Here's how the part is built. I have some questions about the finished solid (model axes, mm). A direction names the side the tool comes from. Coordinates: 2 decimals unless noted, no trailing zeros. Loops run counter-clockwise (first coordinate to the right, second up) from the corner with the lowest first, then second, coordinate; pieces in that order, holes last. Notation, with made-up numbers: (28, -9) - (74, -9) arc R27 ccw to (74, 29) - close; hole circle Ø9 at (10.5, -2). An arc over 180 degrees is marked (long way). Use a Markdown table: item, result.
```python
from build123d import *

# Parameters (mm, degrees)
BOSS_EXTRUDE1_DEPTH = 37
SKETCH2_R           = 1.75
SKETCH2_R_2         = 12.5
SKETCH2_R_3         = 2.75
SKETCH2_R_4         = 2.25
CUT_EXTRUDE1_DEPTH  = 38
SKETCH5_R           = 2.25
CUT_EXTRUDE2_DEPTH  = 38
CUT_EXTRUDE3_DEPTH  = 34
SKETCH7_R           = 4.75
BOSS_EXTRUDE2_DEPTH = 4.5
SKETCH10_W          = 40
SKETCH10_H          = 64
CUT_EXTRUDE4_DEPTH  = 34
SKETCH11_R          = 2.75
CUT_EXTRUDE5_DEPTH  = 8.5
SKETCH12_W          = 15
SKETCH12_H          = 10
SKETCH12_W_2        = 20
SKETCH12_W_3        = 10
BOSS_EXTRUDE3_DEPTH = 34
CUT_EXTRUDE6_DEPTH  = 33
CUT_EXTRUDE8_DEPTH  = 15
CUT_EXTRUDE9_DEPTH  = 15
CUT_EXTRUDE10_DEPTH = 10
CUT_EXTRUDE11_DEPTH = 10
SKETCH20_W          = 6
SKETCH20_H          = 15
CUT_EXTRUDE12_DEPTH = 3


with BuildPart() as part:
    # Sketch1 → Boss-Extrude1 (new body)
    with BuildSketch(Plane.XY):
        with BuildLine():
            Line((-78, 32), (78, 32))
            ThreePointArc((78, 32), (81.535533906, 30.535533906), (83, 27))
            Line((83, 27), (83, -27))
            ThreePointArc((83, -27), (81.535533906, -30.535533906), (78, -32))
            Line((78, -32), (-78, -32))
            ThreePointArc((-78, -32), (-81.535533906, -30.535533906), (-83, -27))
            Line((-83, -27), (-83, 27))
            ThreePointArc((-83, 27), (-81.535533906, 30.535533906), (-78, 32))
        make_face()
    extrude(amount=BOSS_EXTRUDE1_DEPTH)

    # Sketch2 → Cut-Extrude1 (cut, through all)
    with BuildSketch(Plane.XY.offset(37)):
        with Locations((-73.75, 15.75)):
            Circle(SKETCH2_R)
        with Locations((-42.25, 15.75)):
            Circle(SKETCH2_R)
        with Locations((-73.75, -15.75)):
            Circle(SKETCH2_R)
        with Locations((-42.25, -15.75)):
            Circle(SKETCH2_R)
        with Locations((-58, 0)):
            Circle(SKETCH2_R_2)
        with Locations((44, 15)):
            Circle(SKETCH2_R_3)
        with Locations((44, -15)):
            Circle(SKETCH2_R_3)
        with Locations((-18, 0)):
            Circle(SKETCH2_R_3)
        with Locations((64, 0)):
            Circle(SKETCH2_R_4)
    extrude(amount=-CUT_EXTRUDE1_DEPTH, mode=Mode.SUBTRACT)

    # Sketch5 → Cut-Extrude2 (cut, through all)
    with BuildSketch(Plane.XY.offset(37)):
        with Locations((3, 0)):
            Circle(SKETCH5_R)
        with Locations((23, 0)):
            Circle(SKETCH5_R)
    extrude(amount=-CUT_EXTRUDE2_DEPTH, mode=Mode.SUBTRACT)

    # Sketch6 → Cut-Extrude3 (cut)
    with BuildSketch(Plane.XY.offset(37)):
        with BuildLine():
            Line((-78, -29), (78, -29))
            ThreePointArc((78, -29), (79.414213562, -28.414213562), (80, -27))
            Line((80, -27), (80, 27))
            ThreePointArc((80, 27), (79.414213562, 28.414213562), (78, 29))
            Line((78, 29), (-78, 29))
            ThreePointArc((-78, 29), (-79.414213562, 28.414213562), (-80, 27))
            Line((-80, 27), (-80, -27))
            ThreePointArc((-80, -27), (-79.414213562, -28.414213562), (-78, -29))
        make_face()
    extrude(amount=-CUT_EXTRUDE3_DEPTH, mode=Mode.SUBTRACT)

    # Sketch7 → Boss-Extrude2 (add)
    with BuildSketch(Plane.XY.offset(3)):
        with Locations((-18, 0)):
            Circle(SKETCH7_R)
        with Locations((44, -15)):
            Circle(SKETCH7_R)
        with Locations((44, 15)):
            Circle(SKETCH7_R)
    extrude(amount=BOSS_EXTRUDE2_DEPTH)

    # Sketch10 → Cut-Extrude4 (cut)
    with BuildSketch(Plane.XY.offset(37)):
        with Locations((13, 0)):
            Rectangle(SKETCH10_W, SKETCH10_H)
    extrude(amount=-CUT_EXTRUDE4_DEPTH, mode=Mode.SUBTRACT)

    # Sketch11 → Cut-Extrude5 (cut, through all)
    with BuildSketch(Plane.XY.offset(7.5)):
        with Locations((44, -15)):
            Circle(SKETCH11_R)
        with Locations((-18, 0)):
            Circle(SKETCH11_R)
        with Locations((44, 15)):
            Circle(SKETCH11_R)
    extrude(amount=-CUT_EXTRUDE5_DEPTH, mode=Mode.SUBTRACT)

    # Sketch12 → Boss-Extrude3 (add, through all)
    with BuildSketch(Plane.XY.offset(3)):
        with Locations((67.5, -24)):
            Rectangle(SKETCH12_W, SKETCH12_H)
        with Locations((67.5, 24)):
            Rectangle(SKETCH12_W, SKETCH12_H)
        with Locations((70, -11)):
            Rectangle(SKETCH12_W_2, SKETCH12_H)
        with Locations((70, 11)):
            Rectangle(SKETCH12_W_2, SKETCH12_H)
        with Locations((-30, -24)):
            Rectangle(SKETCH12_W_3, SKETCH12_H)
        with Locations((-30, 24)):
            Rectangle(SKETCH12_W_3, SKETCH12_H)
    extrude(amount=BOSS_EXTRUDE3_DEPTH)

    # Sketch14 → Cut-Extrude6 (cut)
    with BuildSketch(Plane.XZ.offset(16)):
        Polygon((80, 37), (60, 37), (60, 3), align=None)
    extrude(amount=-CUT_EXTRUDE6_DEPTH, mode=Mode.SUBTRACT)

    # Sketch16 → Cut-Extrude8 (cut)
    with BuildSketch(Plane(origin=(75, 0, 0), x_dir=(0, 0, -1), z_dir=(1, 0, 0))):
        Polygon((-37, -19), (-3, -19), (-37, -29), align=None)
    extrude(amount=-CUT_EXTRUDE8_DEPTH, mode=Mode.SUBTRACT)

    # Sketch17 → Cut-Extrude9 (cut)
    with BuildSketch(Plane.ZY.offset(-60)):
        Polygon((37, 19), (3, 19), (37, 29), align=None)
    extrude(amount=-CUT_EXTRUDE9_DEPTH, mode=Mode.SUBTRACT)

    # Sketch18 → Cut-Extrude10 (cut)
    with BuildSketch(Plane(origin=(-25, 0, 0), x_dir=(0, 0, -1), z_dir=(1, 0, 0))):
        Polygon((-37, -29), (-37, -19), (-3, -19), align=None)
    extrude(amount=-CUT_EXTRUDE10_DEPTH, mode=Mode.SUBTRACT)

    # Sketch19 → Cut-Extrude11 (cut)
    with BuildSketch(Plane(origin=(-25, 0, 0), x_dir=(0, 0, -1), z_dir=(1, 0, 0))):
        Polygon((-37, 29), (-3, 19), (-37, 19), align=None)
    extrude(amount=-CUT_EXTRUDE11_DEPTH, mode=Mode.SUBTRACT)

    # Sketch20 → Cut-Extrude12 (cut)
    with BuildSketch(Plane.ZY.offset(83)):
        with Locations((30, 0)):
            Rectangle(SKETCH20_W, SKETCH20_H)
    extrude(amount=-CUT_EXTRUDE12_DEPTH, mode=Mode.SUBTRACT)


solid = part.part
```
Q1. I want a section at A-A, the plane x = -42.25. Write out the boundary of the cut face in (y, z), then the cut area to 3 significant figures.
Check values:
| item | result |
|---|---|
| outline | (-32, 0) - (-17.5, 0) - (-17.5, 3) - (-29, 3) - (-29, 37) - (-32, 37) - close; (-14, 0) - (14, 0) - (14, 3) - (-14, 3) - close; (17.5, 0) - (32, 0) - (32, 37) - (29, 37) - (29, 3) - (17.5, 3) - close |
| area | 375 mm^2 |
Q2. Will these pins go through, and if not, where does the flat tip stop? P1, Ø1, axis at x = 47.5, y = 21, coming from the +Z side; P2, Ø2.5, axis at x = -81, y = 3.5, coming from the -Z side.
Check values:
| item | result |
|---|---|
| P1 | z = 3 |
| P2 | z = 0 |
Q3. If we mould it in two halves opening along X, with no side actions, what happens to faces 1 (the face through (-16, -29, 20)), 2 (the face through (-82, 30, 18)), 3 (the face through (82, -30, 18))? For each: pulls with the +X half, pulls with the -X half, needs draft (parallel to the pull), parting line crosses it, or undercut.
Check values:
| item | result |
|---|---|
| face 1 | undercut |
| face 2 | pulls with the -X half |
| face 3 | pulls with the +X half |
Q4. Which directions (+Z, -Z, +X, -X, +Y, -Y) give clear straight access to the entire face, cutting with the end or side of a thin tool? Please do faces 4 (the face through (-35, 26, 12)), 5 (the face through (-82, -7.5, 30)), 6 (the face through (-40.581, -15.224, 1.521)).
Check values:
| item | result |
|---|---|
| face 4 | +Z |
| face 5 | -X |
| face 6 | +Z, -Z |
Q5. I want a section at D-D, the plane x = 44. Write out the boundary of the cut face in (y, z).
Check values:
| item | result |
|---|---|
| outline | (-32, 0) - (-17.75, 0) - (-17.75, 7.5) - (-19.75, 7.5) - (-19.75, 3) - (-29, 3) - (-29, 37) - (-32, 37) - close; (-12.25, 0) - (12.25, 0) - (12.25, 7.5) - (10.25, 7.5) - (10.25, 3) - (-10.25, 3) - (-10.25, 7.5) - (-12.25, 7.5) - close; (17.75, 0) - (32, 0) - (32, 37) - (29, 37) - (29, 3) - (19.75, 3) - (19.75, 7.5) - (17.75, 7.5) - close |
Q6. I want a section at C-C, the plane y = -24.5. Write out the boundary of the cut face in (x, z).
Check values:
| item | result |
|---|---|
| outline | (-83, 0) - (83, 0) - (83, 37) - (80, 37) - (80, 3) - (75, 3) - (75, 21.7) - (60, 21.7) - (60, 3) - (-25, 3) - (-25, 21.7) - (-35, 21.7) - (-35, 3) - (-80, 3) - (-80, 37) - (-83, 37) - close |
Q7. Please list where these lines run through material, in increasing order: L1, parallel to X at y = -21.5, z = 6.5; L2, parallel to Y at x = -42.25, z = 1; L3, parallel to X at y = 24, z = 22. Write a range as from..to.
Check values:
| item | result |
|---|---|
| L1 | -83..-80, -35..-25, 60..75, 80..83 |
| L2 | -32..-17.5, -14..14, 17.5..32 |
| L3 | -83..-80, 80..83 |
Q8. I want a section at B-B, the plane x = -18. Write out the boundary of the cut face in (y, z), then the cut area to 4 significant figures.
Check values:
| item | result |
|---|---|
| outline | (-32, 0) - (-2.75, 0) - (-2.75, 7.5) - (-4.75, 7.5) - (-4.75, 3) - (-29, 3) - (-29, 37) - (-32, 37) - close; (2.75, 0) - (32, 0) - (32, 37) - (29, 37) - (29, 3) - (4.75, 3) - (4.75, 7.5) - (2.75, 7.5) - close |
| area | 397.5 mm^2 |
